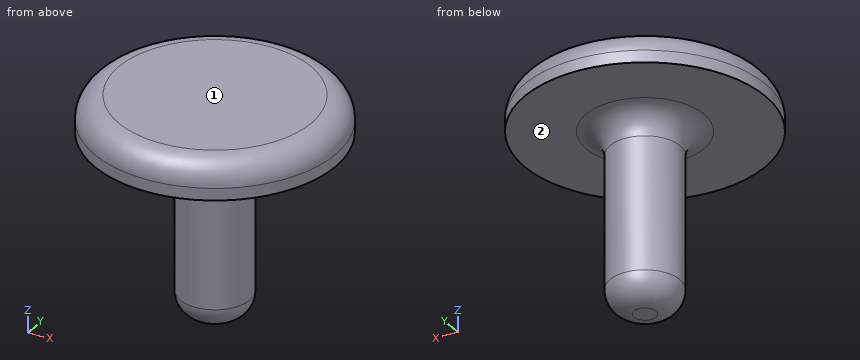
```python
from build123d import *

# Parameters (mm, degrees)
F2_R = 2


with BuildPart() as f1:
    # F0 (on Front) → F1 (revolve)
    with BuildSketch(Plane.XZ):
        Polygon((10, 0), (0, 0), (0, -3), (0, -18), (2.9, -18), (2.9, -3), (10, -3), align=None)
    revolve(axis=Axis((0, 0, -11.278831), (0, 0, -1)))

    # F2
    f2_edges = [f1.edges().sort_by_distance(p)[0] for p in [
        (-2.9, 0, -18),
        (-10, 0, 0),
        (-2.9, 0, -3),
        (2.9, 0, -10.5),
    ]]
    fillet(f2_edges, radius=F2_R)


solid = f1.part
```
Part model, mm, in its own coordinate system. Face numbers are marked on the shaded views. A direction names the side the tool comes from. Coordinates: 2 decimals unless noted, no trailing zeros. Order: outer loops, then holes, each group sorted by start corner. A loop starts at its lowest first (then second) coordinate and runs counter-clockwise, first axis right, second up. Notation, with made-up numbers: (-9, 55.5) - (13, 55.5) arc R12 ccw to (13, 74.5) - close; hole circle Ø6 at (39.25, -38). An arc over 180 degrees is marked (long way). Return JSON: item names as keys, results as strings. Group by question number.
Item 1: Drill centre lines: probe 1 along Z at (x, y) = (3, -4.75); probe 2 along X at (y, z) = (2, -3.25); probe 3 along Z at (x, y) = (-1.25, -0.5). Where is each one in solid material? Low to high. Write a range as from..to.
Item 2: Pin check, flat tips, straight feed: pin 1 (6 mm diameter, centred on x = -5, z = -12, fed in from -Y); pin 2 (4 mm diameter, centred on y = -2.5, z = -9.5, fed in from +X); pin 3 (6 mm diameter, centred on y = 4, z = -6.5, fed in from -X). Stop position of each tip, or through.
Item 3: Cut at A-A (z = -13). List the corners of the cut face in (x, y), plus the area to 3 significant figures.
Item 4: Which spindle directions (+Z, -Z, +X, -X, +Y, -Y) get a long thin tool onto all of the face, cutting with end or side? Do the marked faces 1 and 2. Say none if no direction does.
Check values:
{
 "1": {"probe 1": "z = -3..0", "probe 2": "x = -3.39..3.39", "probe 3": "z = -17.95..0"},
 "2": {"pin 1": "stops at y = -2.1", "pin 2": "stops at x = 2.86", "pin 3": "stops at x = -2.72"},
 "3": {"outline": "circle Ø5.8 at (0, 0)", "area": "26.4 mm2"},
 "4": {"face 1": "+Z, +X, -X, +Y, -Y", "face 2": "-Z"}
}
